from build123d import *

# Parameters (mm, degrees)
SKETCH1_W                  = 80.3
SKETCH1_H                  = 66
BOSS_EXTRUDE1_DEPTH        = 6
F_3_2_3_2_DIAMETER_HOLE1_D = 3.2
FILLET1_R                  = 3
SKETCH4_W                  = 19
SKETCH4_H                  = 34
SKETCH4_W_2                = 31
SKETCH4_H_2                = 16
SKETCH4_W_3                = 7
SKETCH4_H_3                = 7
SKETCH4_W_4                = 13
SKETCH4_H_4                = 17
SKETCH4_W_5                = 40
SKETCH4_H_5                = 19.5
SKETCH4_W_6                = 10
SKETCH4_H_6                = 26
CUT_EXTRUDE1_DEPTH         = 7
CUT_EXTRUDE3_DEPTH         = 7


with BuildPart() as part:
    # Sketch1 → Boss-Extrude1 (new body)
    with BuildSketch(Plane.XY):
        with Locations((40.15, 33)):
            Rectangle(SKETCH1_W, SKETCH1_H)
    extrude(amount=BOSS_EXTRUDE1_DEPTH)

    # Ø3.2 (3.2) Diameter Hole1 (through all)
    with Locations(Plane.XY.offset(6)):
        with Locations((7, 59), (73.3, 59), (73.3, 7), (7, 7)):
            Hole(F_3_2_3_2_DIAMETER_HOLE1_D / 2)

    # Fillet1
    fillet1_edges = [part.edges().sort_by_distance(p)[0] for p in [
        (0, 66, 3),
        (80.3, 66, 3),
        (80.3, 0, 3),
        (0, 0, 3),
    ]]
    fillet(fillet1_edges, radius=FILLET1_R)

    # Sketch4 → Cut-Extrude1 (cut, through all)
    with BuildSketch(Plane.XY.offset(6)):
        with Locations((12.5, 33)):
            Rectangle(SKETCH4_W, SKETCH4_H)
        with Locations((53.8, 55)):
            Rectangle(SKETCH4_W_2, SKETCH4_H_2)
        with Locations((31.5, 53)):
            Rectangle(SKETCH4_W_3, SKETCH4_H_3)
        with Locations((45.8, 32.5)):
            Rectangle(SKETCH4_W_4, SKETCH4_H_4)
        with Locations((45.829355907, 12.75)):
            Rectangle(SKETCH4_W_5, SKETCH4_H_5)
        with Locations((72.3, 24.5)):
            Rectangle(SKETCH4_W_6, SKETCH4_H_6)
    extrude(amount=-CUT_EXTRUDE1_DEPTH, mode=Mode.SUBTRACT)

    # Sketch5 → Cut-Extrude3 (cut, through all)
    with BuildSketch(Plane.XY.offset(6)):
        Polygon((67.3, 11.5), (67.3, 3), (16, 3), (3, 16), (3, 50), (5.071067812, 50), (18.071067812, 63), (38.3, 63), (69.3, 63), (69.3, 47), (38.3, 47), (38.3, 41), (52.3, 41), (52.3, 22.5), (67.3, 22.5), align=None)
    extrude(amount=-CUT_EXTRUDE3_DEPTH, mode=Mode.SUBTRACT)


solid = part.part
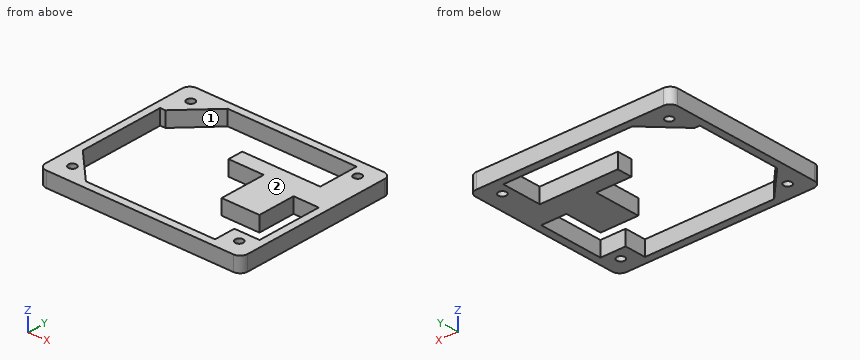
Read the model definition and answer for the solid it produces. Units are mm, in the model's axes. Face numbers are marked on the shaded views. Coordinates: 2 decimals unless noted, no trailing zeros. Loops run counter-clockwise (first coordinate to the right, second up) from the corner with the lowest first, then second, coordinate; pieces in that order, holes last.
Q1. Consider probe 1 along Y at (x, z) = (73.3, 2.2); probe 2 along X at (y, z) = (32.5, 5.5); probe 3 along Y at (x, z) = (68.5, 1). Determine where each line is inside the solid, lowest interval first.
Q2. The part is cut by section A-A on y = 13. Write down the section's boundary in (x, z), and give its area (3 significant figures).
Q3. The part is cut by section D-D on x = 40.5. Write down the section's boundary in (y, z), and give its area (3 significant figures).
Q4. The part is cut by section B-B on x = 73.3. Write down the section's boundary in (y, z), and give its area (3 significant figures).
Q5. The part is cut by section C-C on z = 1.25. Give the number of separate pieces and of enclosed holes in the cut face, and give its area (3 significant figures).
Q6. The mould has two halves that part along X. Classify the marked faces 1 and 2: +X half, -X half, draft (parallel to the pull), parting line (faces both ways), or undercut.
Q7. This flat-tipped pin is pushed along its axis until it touches: pin 1 Ø2.5 at (x, y) = (73.3, 7) entering from -Z. Where does it stop, or does it pass through?
Results below:
1. probe 1: y = 0 to 5.4, 8.6 to 11.5, 37.5 to 57.4, 60.6 to 66
1. probe 2: x = 0 to 3, 52.3 to 67.3, 77.3 to 80.3
1. probe 3: y = 0 to 11.5, 37.5 to 47, 63 to 66
2. outline: (0, 0) - (6, 0) - (6, 6) - (0, 6) - close; (77.3, 0) - (80.3, 0) - (80.3, 6) - (77.3, 6) - close
2. area: 54.0 mm2
3. outline: (0, 0) - (3, 0) - (3, 6) - (0, 6) - close; (41, 0) - (47, 0) - (47, 6) - (41, 6) - close; (63, 0) - (66, 0) - (66, 6) - (63, 6) - close
3. area: 72.0 mm2
4. outline: (0, 0) - (5.4, 0) - (5.4, 6) - (0, 6) - close; (8.6, 0) - (11.5, 0) - (11.5, 6) - (8.6, 6) - close; (37.5, 0) - (57.4, 0) - (57.4, 6) - (37.5, 6) - close; (60.6, 0) - (66, 0) - (66, 6) - (60.6, 6) - close
4. area: 202 mm2
5. separate pieces: 1
5. enclosed holes: 5
5. area: 1,760 mm2
6. face 1: undercut
6. face 2: draft
7. pin 1: passes through
